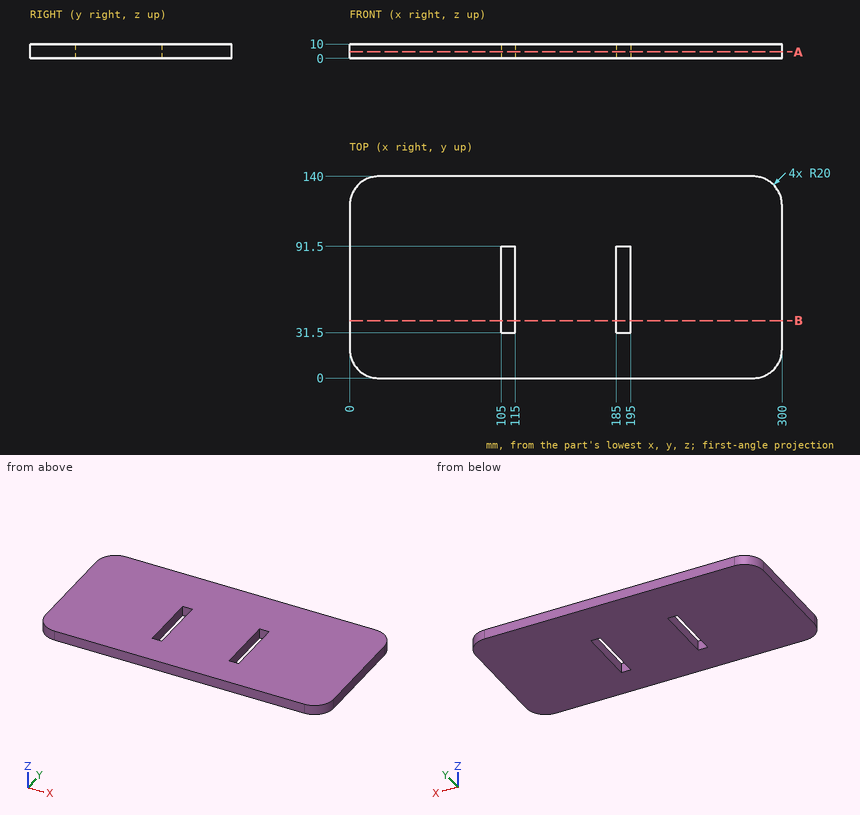
Geometry: see drawing. Coordinates: mm, zero at the bounding-box minimum. Round coordinates to 2 decimals unless told otherwise and drop trailing zeros. Loops run counter-clockwise (first coordinate to the right, second up) from the corner with the lowest first, then second, coordinate; pieces in that order, holes last. Notation, with made-up numbers: (65.25, 3) - (113.25, 3) arc R24 ccw to (113.25, 34) - close; hole circle Ø2 at (10, -23). An arc over 180 degrees is marked (long way). Use CSV: the item, a comma, the result in double quotes.
Q1. Section query A-A, the plane z = 4.5. Output: boundary loops of the cut face in (x, y), then the cut area to 3 significant figures.
Reported:
outline,"(0, 20) arc R20 ccw to (20, 0) - (280, 0) arc R20 ccw to (300, 20) - (300, 120) arc R20 ccw to (280, 140) - (20, 140) arc R20 ccw to (0, 120) - close; hole (105, 31.5) - (115, 31.5) - (115, 91.5) - (105, 91.5) - close; hole (185, 31.5) - (195, 31.5) - (195, 91.5) - (185, 91.5) - close"
area,"40,500 mm^2"
Q2. Ray query, line 1 along X through (y, z) = (37, 2.5); line 2 along Y through (x, z) = (106, 7.25); line 3 along X through (y, z) = (10, 5.5). Return the intervals inside material, ascending.
Reported:
line 1,"0 to 105, 115 to 185, 195 to 300"
line 2,"0 to 31.5, 91.5 to 140"
line 3,"2.68 to 297.32"
Q3. Section query B-B, the plane y = 40. Output: boundary loops of the cut face in (x, z), then the cut area to 3 significant figures.
Reported:
outline,"(0, 0) - (105, 0) - (105, 10) - (0, 10) - close; (115, 0) - (185, 0) - (185, 10) - (115, 10) - close; (195, 0) - (300, 0) - (300, 10) - (195, 10) - close"
area,"2,800 mm^2"
